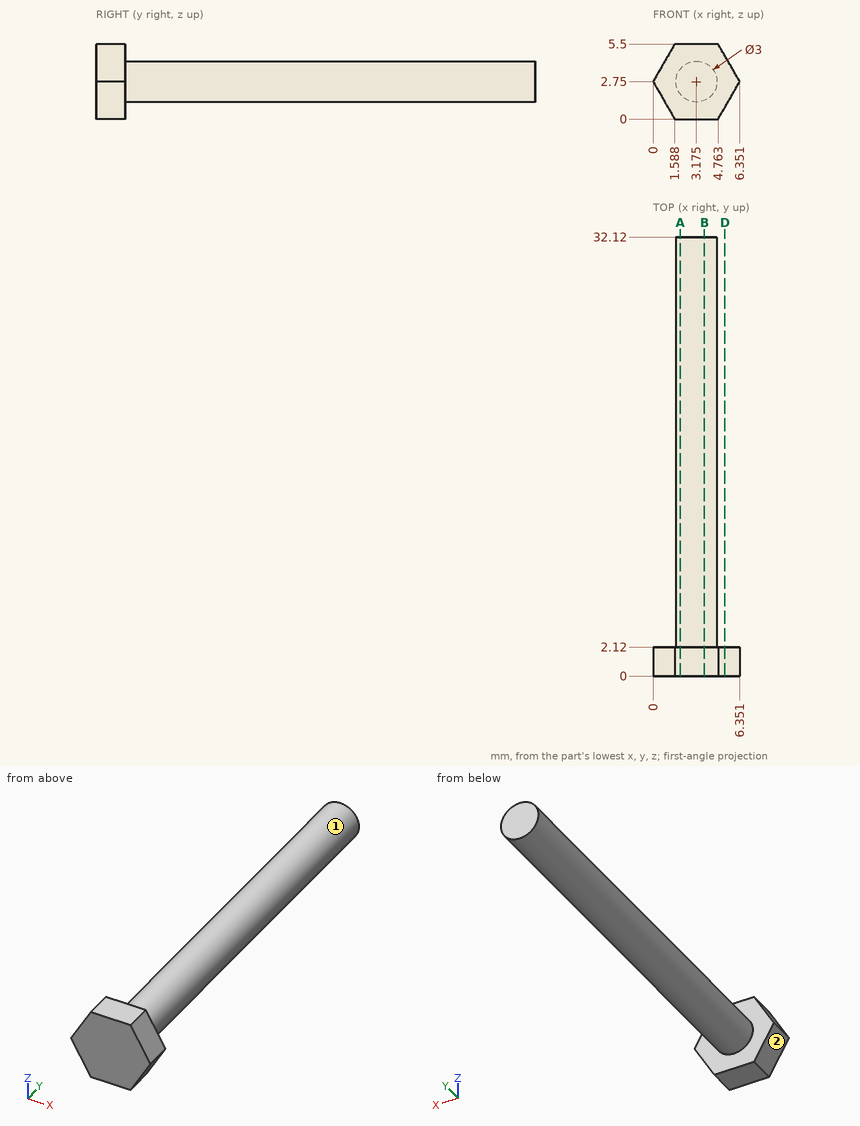
Job drawing, mm, ordinate dimensions from the low corner. One solid piece. A direction names the side the tool comes from. Give positions to 0.01 mm unless a question says otherwise; leave off trailing zeros. Write each loop counter-clockwise with the first axis right and the second up, starting at its lowest first coordinate (ties: lowest second). Pieces come first, ordered by that corner, then holes. Notation, with made-up numbers: (55, 77) - (92, 77) arc R16 ccw to (92, 90) - close; hole circle Ø4 at (-33.5, -4). An arc over 180 degrees is marked (long way). Answer as CSV lines item,"result".
1. Pin check, flat tips, straight feed: pin 1 (1 mm diameter, centred on x = 0.5, y = 14, fed in from -Z); pin 2 (1 mm diameter, centred on y = 8, z = 2.5, fed in from -X) (1 decimal); pin 3 (1 mm diameter, centred on x = 4, y = 4, fed in from -Z) (1 decimal). Stop position of each tip, or through.
Responses:
pin 1,"passes through"
pin 2,"stops at x = 1.7"
pin 3,"stops at z = 1.3"
2. Band-saw the part on D-D (x = 5.25). Write the cut outline in (y, z).
Responses:
outline,"(0, 0.84) - (2.12, 0.84) - (2.12, 4.66) - (0, 4.66) - close"
3. Drill centre lines: L1, parallel to Y at x = 5, z = 4.9; L2, parallel to Z at x = 3.25, y = 5; L3, parallel to X at y = 17, z = 3 (1 decimal). Where is each one in solid material? Low to high. Write a range as [from, to].
Responses:
L1,"y = [0, 2.12]"
L2,"z = [1.25, 4.25]"
L3,"x = [1.7, 4.7]"
4. Band-saw the part on A-A (x = 2). Write the cut outline in (y, z).
Responses:
outline,"(0, 0) - (2.12, 0) - (2.12, 1.82) - (32.12, 1.82) - (32.12, 3.68) - (2.12, 3.68) - (2.12, 5.5) - (0, 5.5) - close"
5. 3-axis set-ups, long thin cutter, end or side, ignore diameter. For the marked faces 1 and 2: which of +Z, -Z, +X, -X, +Y, -Y reach the whole face in a straight line?
Responses:
face 1,"+Y"
face 2,"-Z, -X, +Y, -Y"
6. Band-saw the part on B-B (x = 3.75). Write the cut outline in (y, z) (1 decimal).
Responses:
outline,"(0, 0) - (2.1, 0) - (2.1, 1.4) - (32.1, 1.4) - (32.1, 4.1) - (2.1, 4.1) - (2.1, 5.5) - (0, 5.5) - close"
